Build history of the part. All positions in model axes, mm. A direction names the side the tool comes from. Round coordinates to 2 decimals unless told otherwise and drop trailing zeros. Write each loop counter-clockwise with the first axis right and the second up, starting at its lowest first coordinate (ties: lowest second). Pieces come first, ordered by that corner, then holes.
Item 1: 3-axis set-ups, long thin cutter, end or side, ignore diameter. For faces 4 (the flat face through (12.5, 0, 7)), 5 (the cylindrical face through (7.99, 7.24, 20.18)), 6 (the flat face through (-12.5, 0, 7)), 7 (the cylindrical face through (-0.07, 6.4, -9.88)), 8 (the cylindrical face through (-2.87, -0.2, 6.93)): which of +Z, -Z, +X, -X, +Y, -Y reach the whole face in a straight line?
Item 2: Drop flat-ended pins along their axis: pin 1 Ø12 at (y, z) = (-11, -3) entering from +X; pin 2 Ø4 at (x, y) = (7, -8) entering from -Z; pin 3 Ø11 at (x, y) = (-21.5, -3) entering from -Z. Give the stop position or say it passes through.
Item 3: Band-saw the part on A-A, the plane x = 23.5. Write the cut outline in (y, z).
Item 4: Band-saw the part on D-D, the plane x = -10. Write the cut outline in (y, z), then the cut area to 3 significant figures.
Item 5: Mould opens along Y. For faces 1 (the cylindrical face through (-24.24, -7.58, 23.48)), 2 (the cylindrical face through (-22.76, 7.58, 23.48)), 3 (the flat face through (-14.965, -0.196, 17.609)) say: +Y half, -Y half, draft (parallel to the pull), parting line (faces both ways), or undercut.
Item 6: Band-saw the part on C-C, the plane z = -6. Write the cut outline in (x, y).
Item 7: Wall check: probe 1 along Y at (x, z) = (-23.5, 23); probe 2 along Y at (x, z) = (7, 20.5); probe 3 along X at (y, z) = (8, 22.5). Give the ranges that are in metal, low to high.
Item 8: Band-saw the part on B-B, the plane y = -0.25. Write the cut outline in (x, z).
```python
from build123d import *
from OCP.BRepFilletAPI import BRepFilletAPI_MakeChamfer

# Parameters (mm, degrees)
SKETCH_1_R             = 7.5
EXTRUDE_1_DEPTH        = 14
SKETCH_7_R             = 1.6
CUT_EXTRUDE_2_DEPTH    = 32.260998065
HOLE_WIZARD_M3_1_D     = 2.5
HOLE_WIZARD_M3_1_DEPTH = 9.5
HOLE_WIZARD_M3_1_TIP   = 0.751075774
SKETCH_9_W             = 3
SKETCH_9_H             = 28
EXTRUDE_2_DEPTH        = 15
SKETCH_10_R            = 1.6
CUT_EXTRUDE_3_DEPTH    = 47.287147349
CHAMFER_1_SIZE         = 5
CHAMFER_1_SIZE2        = 8.660254038


with BuildPart() as part:
    # 草图1 → 凸台-拉伸1 (new, symmetric)
    with BuildSketch(Plane(origin=(0, 0, 0), x_dir=(1, 0, 0), z_dir=(0, 1, 0))):
        with BuildLine():
            Line((-12.5, -25), (12.5, -25))
            Line((12.5, -25), (12.5, 0))
            ThreePointArc((12.5, 0), (0, 12.5), (-12.5, 0))
            Line((-12.5, 0), (-12.5, -25))
        make_face()
        with Locations(Location((0, 0, 0), (0, 0, 270))):
            Circle(SKETCH_1_R, mode=Mode.SUBTRACT)
    extrude(amount=EXTRUDE_1_DEPTH, both=True)

    # 草图7 → 切除-拉伸2 (cut, through all)
    with BuildSketch(Plane.XY):
        with Locations(Location((0, -8, 0), (0, 0, 90))):
            Circle(SKETCH_7_R)
        with Locations(Location((0, 8, 0), (0, 0, 90))):
            Circle(SKETCH_7_R)
    extrude(amount=-CUT_EXTRUDE_2_DEPTH, mode=Mode.SUBTRACT)

    # M3 螺纹孔1
    with Locations(Plane(origin=(-7, -8, 25), x_dir=(1, 0, 0), z_dir=(0, 0, 1))):
        with Locations((0, 0), (14, 0), (14, 16), (0, 16)):
            Hole(HOLE_WIZARD_M3_1_D / 2, depth=HOLE_WIZARD_M3_1_DEPTH)
            with Locations((0, 0, -(HOLE_WIZARD_M3_1_DEPTH + HOLE_WIZARD_M3_1_TIP / 2))):  # 118° drill point
                Cone(0, HOLE_WIZARD_M3_1_D / 2, HOLE_WIZARD_M3_1_TIP, mode=Mode.SUBTRACT)

    # 草图9 → 凸台-拉伸2 (add)
    with BuildSketch(Plane(origin=(12.5, 0, 0), x_dir=(0, 0, -1), z_dir=(1, 0, 0))):
        with Locations((-23.5, 0)):
            Rectangle(SKETCH_9_W, SKETCH_9_H)
    extrude_2 = extrude(amount=EXTRUDE_2_DEPTH)

    # 草图10 → 切除-拉伸3 (cut, through all)
    with BuildSketch(Plane(origin=(0, 0, 22), x_dir=(-1, 0, 0), z_dir=(0, 0, -1))):
        with Locations((-23.5, 9)):
            Circle(SKETCH_10_R)
        with Locations(Location((-23.5, -9, 0), (0, 0, 180))):
            Circle(SKETCH_10_R)
    cut_extrude_3 = extrude(amount=-CUT_EXTRUDE_3_DEPTH, mode=Mode.SUBTRACT)

    # 镜向6: 凸台-拉伸2, 切除-拉伸3 across plane
    add(extrude_2.mirror(Plane(origin=(0, 0, 0), x_dir=(0, 0, 1), z_dir=(1, 0, 0))))
    add(cut_extrude_3.mirror(Plane(origin=(0, 0, 0), x_dir=(0, 0, 1), z_dir=(1, 0, 0))), mode=Mode.SUBTRACT)

    # 倒角1: one chamfer whose edges measure the first distance from different faces: ONE call of the kernel's chamfer builder (chamfer() names one face for all edges)
    chamfer_1_edges_1 = [part.edges().sort_by_distance(p)[0] for p in [
        (12.5, 0, 22),
    ]]
    chamfer_1_side_1 = [part.faces().sort_by_distance(p)[0] for p in [
        (19.860620839, 0, 22),
    ]]
    chamfer_1_edges_2 = [part.edges().sort_by_distance(p)[0] for p in [
        (-12.5, 0, 22),
    ]]
    chamfer_1_side_2 = [part.faces().sort_by_distance(p)[0] for p in [
        (-19.860620839, 0, 22),
    ]]
    chamfer_1 = BRepFilletAPI_MakeChamfer(part.part.solid().wrapped)
    for e in chamfer_1_edges_1:
        chamfer_1.Add(CHAMFER_1_SIZE, CHAMFER_1_SIZE2, e.wrapped, chamfer_1_side_1[0].wrapped)  # the first distance lies on this face
    for e in chamfer_1_edges_2:
        chamfer_1.Add(CHAMFER_1_SIZE, CHAMFER_1_SIZE2, e.wrapped, chamfer_1_side_2[0].wrapped)  # the first distance lies on this face
    add(Compound.cast(chamfer_1.Shape()), mode=Mode.REPLACE)


solid = part.part
```
Results:
1. face 4: -Z, +X, +Y, -Y
1. face 5: +Z
1. face 6: -Z, -X, +Y, -Y
1. face 7: -Z
1. face 8: +Y, -Y
2. pin 1: stops at x = 12.5
2. pin 2: stops at z = -11.46
2. pin 3: stops at z = 19.4
3. outline: (-14, 22) - (-10.6, 22) - (-10.6, 25) - (-14, 25) - close; (-7.4, 22) - (7.4, 22) - (7.4, 25) - (-7.4, 25) - close; (10.6, 22) - (14, 22) - (14, 25) - (10.6, 25) - close
4. outline: (-14, -7.5) - (14, -7.5) - (14, 25) - (-14, 25) - close
4. area: 910 mm2
5. face 1: undercut
5. face 2: undercut
5. face 3: draft
6. outline: (-10.97, -14) - (-4.5, -14) - (-4.5, 14) - (-10.97, 14) - close; (4.5, -14) - (10.97, -14) - (10.97, 14) - (4.5, 14) - close
7. probe 1: y = -14 to -10.6, -7.4 to 7.4, 10.6 to 14
7. probe 2: y = -14 to -9.25, -6.75 to 6.75, 9.25 to 14
7. probe 3: x = -27.5 to -24.75, -22.25 to -8.25, -5.75 to 5.75, 8.25 to 22.25, 24.75 to 27.5
8. outline: (-27.5, 22) - (-17.5, 22) - (-12.5, 13.34) - (-12.5, 0) arc R12.5 ccw to (12.5, 0) - (12.5, 13.34) - (17.5, 22) - (27.5, 22) - (27.5, 25) - (-27.5, 25) - close; hole circle Ø15 at (0, 0)
